Read the model definition and answer for the solid it produces. Units are mm, in the model's axes. Face numbers are marked on the shaded views. Coordinates: 2 decimals unless noted, no trailing zeros. Order: outer loops, then holes, each group sorted by start corner. A loop starts at its lowest first (then second) coordinate and runs counter-clockwise, first axis right, second up. Notation, with made-up numbers: M 11.5,45 L 36.5,45 A36 cw 36.5,84 Z; hole C 2.5,39 d2. An arc over 180 degrees is marked long. Use a Markdown table: item, result. Add a question column.
1) Find section C-C on x = -38. Write down the section's boundary in (y, z).
2) The mould has two halves that part along Z. Classify the marked faces 1, 2, 3 and 4: released by +Z, released by -Z, zero draft, split by the parting line, or undercut.
3) Find section A-A on y = 10.5. Write down the section's boundary in (x, z).
4) Find section D-D on x = 37. Write down the section's boundary in (y, z), plus the area to 3 significant figures.
5) Find the intervals of material crossed by probe 1 along Z at (x, y) = (20, 14); probe 2 along Y at (x, z) = (17, -10.8); probe 3 along X at (y, z) = (17, 11.75), in increasing order. Write a range as [from, to].
6) Each of these flat-tipped pins is pushed along its axis until it touches: pin 1 Ø4 at (x, z) = (-26.5, -3.5) entering from +Y; pin 2 Ø4 at (x, y) = (-0.42, 36.94) entering from -Z. Where does it stop, or does it pass through?
7) Find section B-B on x = -14. Write down the section's boundary in (y, z).
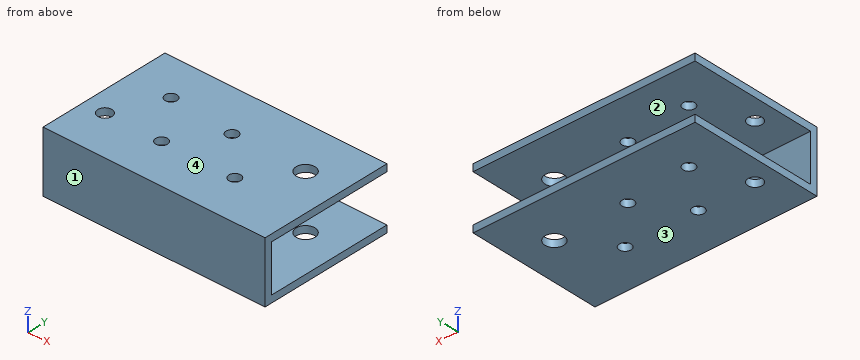
from build123d import *

# Parameters (mm, degrees)
SKETCH_1_W          = 94
SKETCH_1_H          = 26
EXTRUDE_1_DEPTH     = 3
SKETCH_2_W          = 94
SKETCH_2_H          = 3
EXTRUDE_2_DEPTH     = 54
SKETCH_3_R          = 3
SKETCH_3_R_2        = 2.5
SKETCH_3_R_3        = 4
CUT_EXTRUDE_1_DEPTH = 79.319856997


with BuildPart() as part:
    # 스케치1 → 보스-돌출1 (new body)
    with BuildSketch(Plane(origin=(0, 0, 0), x_dir=(1, 0, 0), z_dir=(0, 1, 0))):
        Rectangle(SKETCH_1_W, SKETCH_1_H)
    extrude(amount=EXTRUDE_1_DEPTH)

    # 스케치2 → 보스-돌출2 (add)
    with BuildSketch(Plane(origin=(0, 3, 0), x_dir=(1, 0, 0), z_dir=(0, 1, 0))):
        with Locations((0, 11.5)):
            Rectangle(SKETCH_2_W, SKETCH_2_H)
        with Locations((0, -11.5)):
            Rectangle(SKETCH_2_W, SKETCH_2_H)
    extrude(amount=EXTRUDE_2_DEPTH)

    # 스케치3 → 컷-돌출1 (cut, through all)
    with BuildSketch(Plane.XY.offset(13)):
        with Locations((-38, 19)):
            Circle(SKETCH_3_R)
        with Locations((17, 19)):
            Circle(SKETCH_3_R_2)
        with Locations((-14, 19)):
            Circle(SKETCH_3_R_2)
        with Locations((-28.473958333, 39.383928232)):
            Circle(SKETCH_3_R_2)
        with Locations((-0.415322581, 36.936179621)):
            Circle(SKETCH_3_R_2)
        with Locations((31, 36.613914954)):
            Circle(SKETCH_3_R_3)
    extrude(amount=-CUT_EXTRUDE_1_DEPTH, mode=Mode.SUBTRACT)


solid = part.part
Check result:
| question | item | result |
|---|---|---|
| 1 | outline | M 0,-13 L 16,-13 L 16,-10 L 3,-10 L 3,10 L 16,10 L 16,13 L 0,13 Z; M 22,-13 L 57,-13 L 57,-10 L 22,-10 Z; M 22,10 L 57,10 L 57,13 L 22,13 Z |
| 2 | face 1 | zero draft |
| 2 | face 2 | undercut |
| 2 | face 3 | released by -Z |
| 2 | face 4 | released by +Z |
| 3 | outline | M -47,-13 L 47,-13 L 47,-10 L -47,-10 Z; M -47,10 L 47,10 L 47,13 L -47,13 Z |
| 4 | outline | M 0,-13 L 57,-13 L 57,-10 L 3,-10 L 3,10 L 57,10 L 57,13 L 0,13 Z |
| 4 | area | 402 mm2 |
| 5 | probe 1 | z = [-13, -10], [10, 13] |
| 5 | probe 2 | y = [0, 16.5], [21.5, 57] |
| 5 | probe 3 | x = [-47, -40.24], [-35.76, -15.5], [-12.5, 15.5], [18.5, 47] |
| 6 | pin 1 | stops at y = 3 |
| 6 | pin 2 | passes through |
| 7 | outline | M 0,-13 L 16.5,-13 L 16.5,-10 L 3,-10 L 3,10 L 16.5,10 L 16.5,13 L 0,13 Z; M 21.5,-13 L 57,-13 L 57,-10 L 21.5,-10 Z; M 21.5,10 L 57,10 L 57,13 L 21.5,13 Z |
